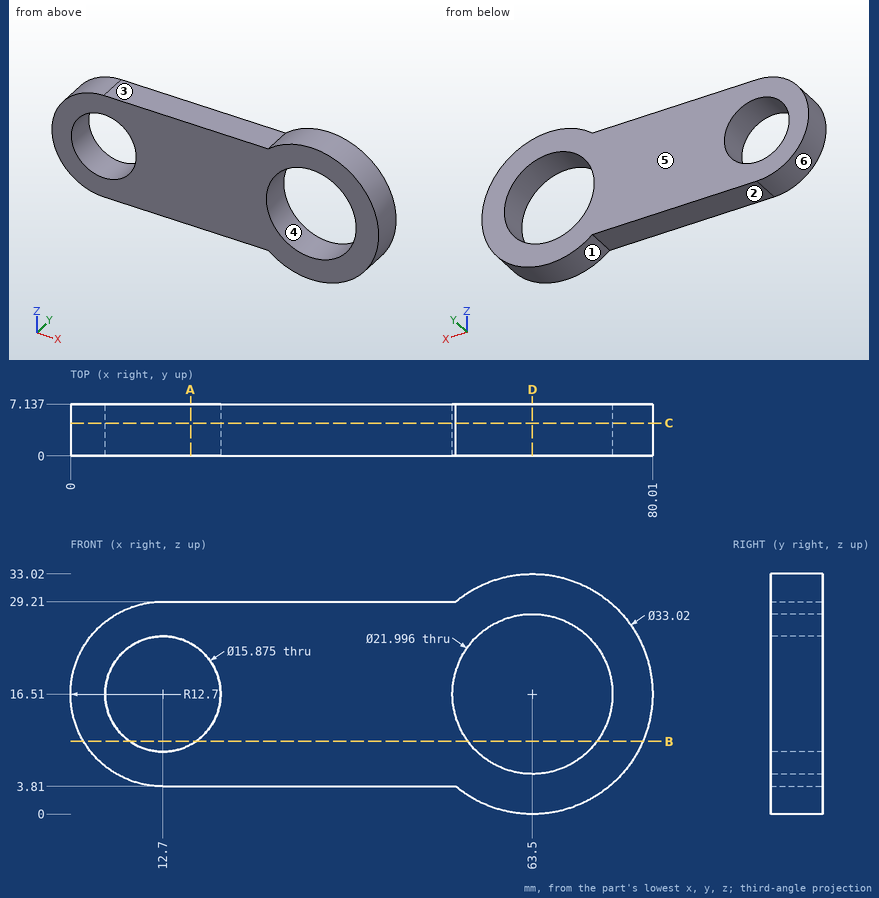
Source: three-view drawing plus pictorial views. Frame: mm from the lowest corner of the part. A direction names the side the tool comes from. Give positions to 0.01 mm unless a question says otherwise; leave off trailing zeros. Write each loop counter-clockwise with the first axis right and the second up, starting at its lowest first coordinate (ties: lowest second). Pieces come first, ordered by that corner, then holes.
(1) Access query for the marked faces 1, 2 and 3. Directions: +Z, -Z, +X, -X, +Y, -Y. A direction counts if a zero-diameter tool reaches every point of the face in a straight line with its end or side. Return the directions, or none.
(2) Cut plane A-A, the plane x = 16.5. Return loops of the section in (y, z).
(3) Ray query, line 1 (X direction, y = 2.5, z = 16); line 2 (Z direction, x = 63.5, y = 5.5); line 3 (X direction, y = 3.25, z = 13.5) (1 decimal). Return the intervals inside material, ascending.
(4) Mould query, pull axis Z, two halves, no side actions, for the marked faces 4, 5 and 6. Classes: released by +Z, released by -Z, zero draft, split by the parting line, or undercut.
(5) Cut plane C-C, the plane y = 4.5. Give the number of separate pieces and of enclosed holes in the cut face, then the cut area to 3 significant figures.
(6) Cut plane B-B, the plane z = 10. Return loops of the section in (x, y) (1 decimal), then the cut area to 3 significant figures.
(7) First-contact query: P1, Ø1, axis at y = 4, z = 8.5, coming from the +X side; P2, Ø4, axis at x = 51.5, y = 5, coming from the -Z side; P3, Ø17.5, axis at x = 63.5, z = 16.51, coming from the -Y side; P4, Ø5, axis at x = 72, z = 23, coming from the -Y side. Flat tips, straight axial feed; report the tip coordinate or a pass-through.
(8) Cut plane D-D, the plane x = 63.5. Return loops of the section in (y, z).
Values follow:
1. face 1: +Y, -Y
1. face 2: -Z, -X, +Y, -Y
1. face 3: +Z, -X, +Y, -Y
2. outline: (0, 3.81) - (7.14, 3.81) - (7.14, 9.54) - (0, 9.54) - close; (0, 23.48) - (7.14, 23.48) - (7.14, 29.21) - (0, 29.21) - close
3. line 1: x = 0.01 to 4.78, 20.62 to 52.51, 74.49 to 80
3. line 2: z = 0 to 5.51, 27.51 to 33.02
3. line 3: x = 0.4 to 5.4, 20 to 52.9, 74.1 to 79.7
4. face 4: undercut
4. face 5: zero draft
4. face 6: split by the parting line
5. separate pieces: 1
5. enclosed holes: 2
5. area: 1,450 mm2
6. outline: (1.8, 0) - (8.2, 0) - (8.2, 7.1) - (1.8, 7.1) - close; (17.2, 0) - (54.6, 0) - (54.6, 7.1) - (17.2, 7.1) - close; (72.4, 0) - (78.7, 0) - (78.7, 7.1) - (72.4, 7.1) - close
6. area: 357 mm2
7. P1: stops at x = 78.2
7. P2: stops at z = 3.37
7. P3: passes through
7. P4: stops at y = 0
8. outline: (0, 0) - (7.14, 0) - (7.14, 5.51) - (0, 5.51) - close; (0, 27.51) - (7.14, 27.51) - (7.14, 33.02) - (0, 33.02) - close
